Input: part model. Units: mm. Frame: model coordinates. Round coordinates to 2 decimals unless told otherwise and drop trailing zeros. Loops run counter-clockwise (first coordinate to the right, second up) from the corner with the lowest first, then second, coordinate; pieces in that order, holes last. Notation, with made-up numbers: (15, 42) -> (59, 42) arc R29 cw to (59, 79) -> close; hole circle Ø11 at (-36, 21.25). An arc over 180 degrees is marked (long way). Answer as a JSON object with one key per item and string values.
```python
from build123d import *

# Parameters (mm, degrees)
EXTRUDE_2_DEPTH = 3


with BuildPart() as part:
    # Эскиз3 → Бобышка-Вытянуть2 (new body)
    with BuildSketch(Plane(origin=(0, 0, 0), x_dir=(1, 0, 0), z_dir=(0, 1, 0))):
        Polygon((-75, 27.5), (-75, 30.5), (-65, 30.5), (-65, 27.5), (-55, 27.5), (-55, 30.5), (-45, 30.5), (-45, 27.5), (-35, 27.5), (-35, 30.5), (-25, 30.5), (-25, 27.5), (-15, 27.5), (-15, 30.5), (-5, 30.5), (-5, 27.5), (5, 27.5), (5, 30.5), (15, 30.5), (15, 27.5), (25, 27.5), (25, 30.5), (35, 30.5), (35, 27.5), (45, 27.5), (45, 30.5), (55, 30.5), (55, 27.5), (65, 27.5), (65, 30.5), (75, 30.5), (75, 27.5), (85, 27.5), (85, 30.5), (95, 30.5), (95, 27.5), (110, 27.5), (113, 27.5), (113, 17.5), (110, 17.5), (110, 7.5), (113, 7.5), (113, -7.5), (110, -7.5), (110, -17.5), (113, -17.5), (113, -27.5), (110, -27.5), (95, -27.5), (95, -30.5), (85, -30.5), (85, -27.5), (75, -27.5), (75, -30.5), (65, -30.5), (65, -27.5), (55, -27.5), (55, -30.5), (45, -30.5), (45, -27.5), (35, -27.5), (35, -30.5), (25, -30.5), (25, -27.5), (15, -27.5), (15, -30.5), (5, -30.5), (5, -27.5), (-5, -27.5), (-5, -30.5), (-15, -30.5), (-15, -27.5), (-25, -27.5), (-25, -30.5), (-35, -30.5), (-35, -27.5), (-45, -27.5), (-45, -30.5), (-55, -30.5), (-55, -27.5), (-65, -27.5), (-65, -30.5), (-75, -30.5), (-75, -27.5), (-85, -27.5), (-85, -30.5), (-95, -30.5), (-95, -27.5), (-110, -27.5), (-110, -17.5), (-113, -17.5), (-113, -7.5), (-110, -7.5), (-110, 7.5), (-113, 7.5), (-113, 17.5), (-110, 17.5), (-110, 27.5), (-95, 27.5), (-95, 30.5), (-85, 30.5), (-85, 27.5), align=None)
    extrude(amount=EXTRUDE_2_DEPTH)


solid = part.part
```
1) Contact query for flat-ended pins moving along their axis: P1, Ø1.5, axis at y = 2, z = -29.5, coming from the -X side; P2, Ø1.5, axis at y = 1, z = -28.5, coming from the +X side; P3, Ø12, axis at x = 59.5, z = 21.5, coming from the -Y side; P4, Ø1.5, axis at x = -105.5, y = 2, coming from the +Z side. Output: stop coordinate, or through.
Output:
{"P1": "stops at x = -95", "P2": "stops at x = 95", "P3": "stops at y = 0", "P4": "stops at z = 27.5"}
2) Section A-A, the plane x = 78.5. Output: boundary loops of the cut face in (y, z), plus the area to 3 significant figures.
Output:
{"outline": "(0, -27.5) -> (3, -27.5) -> (3, 27.5) -> (0, 27.5) -> close", "area": "165 mm^2"}
3) Ray query, probe 1 along X at (y, z) = (1.6, -4); probe 2 along Z at (x, y) = (-101.5, 0.6); probe 3 along X at (y, z) = (0.4, 11.5). Return the intervals inside material, ascending.
Output:
{"probe 1": "x = -110 to 113", "probe 2": "z = -27.5 to 27.5", "probe 3": "x = -113 to 110"}
